The listing builds one solid part. Answer for the finished solid, in the listing's coordinates (mm). A direction names the side the tool comes from. Coordinates: 2 decimals unless noted, no trailing zeros. Write each loop counter-clockwise with the first axis right and the second up, starting at its lowest first coordinate (ties: lowest second). Pieces come first, ordered by that corner, then holes.
from build123d import *

# Parameters (mm, degrees)
SKETCH1_W           = 16
SKETCH1_H           = 37
SKETCH1_W_2         = 13
SKETCH1_H_2         = 34
BOSS_EXTRUDE1_DEPTH = 5
SKETCH2_W           = 16
SKETCH2_H           = 37
BOSS_EXTRUDE2_DEPTH = 1
SKETCH3_W           = 10
SKETCH3_H           = 5
CUT_EXTRUDE1_DEPTH  = 21
SKETCH4_W           = 7
SKETCH4_H           = 2.2
CUT_EXTRUDE2_DEPTH  = 2
SKETCH5_R           = 2.5
CUT_EXTRUDE3_DEPTH  = 2
SKETCH6_W           = 10
SKETCH6_H           = 3
CUT_EXTRUDE4_DEPTH  = 2
CHAMFER1_SIZE       = 1
SKETCH7_W           = 12
SKETCH7_H           = 1
BOSS_EXTRUDE3_DEPTH = 6
SKETCH8_W           = 12
SKETCH8_H           = 1
BOSS_EXTRUDE4_DEPTH = 6
FILLET1_R           = 2
SKETCH9_R           = 1.5
CUT_EXTRUDE5_DEPTH  = 6
SKETCH12_R          = 4
CUT_EXTRUDE6_DEPTH  = 0.8
CHAMFER2_SIZE       = 1.5


with BuildPart() as part:
    # Sketch1 → Boss-Extrude1 (new body)
    with BuildSketch(Plane(origin=(0, 0, 0), x_dir=(1, 0, 0), z_dir=(0, 1, 0))):
        Rectangle(SKETCH1_W, SKETCH1_H)
        Rectangle(SKETCH1_W_2, SKETCH1_H_2, mode=Mode.SUBTRACT)
    extrude(amount=BOSS_EXTRUDE1_DEPTH)

    # Sketch2 → Boss-Extrude2 (add)
    with BuildSketch(Plane.XZ):
        Rectangle(SKETCH2_W, SKETCH2_H)
    extrude(amount=BOSS_EXTRUDE2_DEPTH)

    # Sketch3 → Cut-Extrude1 (cut)
    with BuildSketch(Plane(origin=(8, 0, 0), x_dir=(0, 0, -1), z_dir=(1, 0, 0))):
        with Locations((-11.5, 2.5)):
            Rectangle(SKETCH3_W, SKETCH3_H)
    extrude(amount=-CUT_EXTRUDE1_DEPTH, mode=Mode.SUBTRACT)

    # Sketch4 → Cut-Extrude2 (cut)
    with BuildSketch(Plane.ZY.offset(8)):
        with Locations((-2.4, 3.9)):
            Rectangle(SKETCH4_W, SKETCH4_H)
    extrude(amount=-CUT_EXTRUDE2_DEPTH, mode=Mode.SUBTRACT)

    # Sketch5 → Cut-Extrude3 (cut)
    with BuildSketch(Plane.XY.offset(18.5)):
        with Locations((0, 5.5)):
            Circle(SKETCH5_R)
    extrude(amount=-CUT_EXTRUDE3_DEPTH, mode=Mode.SUBTRACT)

    # Sketch6 → Cut-Extrude4 (cut)
    with BuildSketch(Plane.XY.offset(-17)):
        with Locations((0, 3.5)):
            Rectangle(SKETCH6_W, SKETCH6_H)
    extrude(amount=-CUT_EXTRUDE4_DEPTH, mode=Mode.SUBTRACT)

    # Chamfer1
    chamfer1_edges = [part.edges().sort_by_distance(p)[0] for p in [
        (0, 2, -18.5),
    ]]
    chamfer(chamfer1_edges, length=CHAMFER1_SIZE)

    # Sketch7 → Boss-Extrude3 (add)
    with BuildSketch(Plane(origin=(8, 0, 0), x_dir=(0, 0, -1), z_dir=(1, 0, 0))):
        with Locations((-12.5, -0.5)):
            Rectangle(SKETCH7_W, SKETCH7_H)
    extrude(amount=BOSS_EXTRUDE3_DEPTH)

    # Sketch8 → Boss-Extrude4 (add)
    with BuildSketch(Plane.ZY.offset(8)):
        with Locations((12.5, -0.5)):
            Rectangle(SKETCH8_W, SKETCH8_H)
    extrude(amount=BOSS_EXTRUDE4_DEPTH)

    # Fillet1
    fillet1_edges = [part.edges().sort_by_distance(p)[0] for p in [
        (14, -0.5, 18.5),
        (14, -0.5, 6.5),
        (-14, -0.5, 18.5),
        (-14, -0.5, 6.5),
    ]]
    fillet(fillet1_edges, radius=FILLET1_R)

    # Sketch9 → Cut-Extrude5 (cut)
    with BuildSketch(Plane(origin=(0, 0, 0), x_dir=(1, 0, 0), z_dir=(0, 1, 0))):
        with Locations(Location((-9.25, -11.2, 0), (0, 0, 270))):
            Circle(SKETCH9_R)
        with Locations(Location((9.75, -11.2, 0), (0, 0, 270))):
            Circle(SKETCH9_R)
    extrude(amount=-CUT_EXTRUDE5_DEPTH, mode=Mode.SUBTRACT)

    # Sketch12 → Cut-Extrude6 (cut)
    with BuildSketch(Plane(origin=(0, 0, 17), x_dir=(-1, 0, 0), z_dir=(0, 0, -1))):
        with Locations((0, 5.5)):
            Circle(SKETCH12_R)
    extrude(amount=-CUT_EXTRUDE6_DEPTH, mode=Mode.SUBTRACT)

    # Chamfer2
    chamfer2_edges = [part.edges().sort_by_distance(p)[0] for p in [
        (6.5, 2.5, 6.5),
        (-6.5, 2.5, 6.5),
    ]]
    chamfer(chamfer2_edges, length=CHAMFER2_SIZE - 0.0001)  # a hair under: the kernel refuses the full size


solid = part.part
1. Flat-ended cylindrical pins translate along their axes: P1, Ø8.5, axis at x = 0, z = -3.5, coming from the +Y side; P2, Ø1.8, axis at y = 1.5, z = -7.5, coming from the +X side; P3, Ø1.1, axis at x = -10.5, y = -0.5, coming from the -Z side. Find the tip coordinate at first contact, or state that the pin passes through.
Results found:
P1: stops at y = 0
P2: stops at x = 8
P3: stops at z = 6.5
2. Find the intervals of material crossed by L1, parallel to X at y = -0.25, z = 11.2; L2, parallel to X at y = 0.25, z = -2.5; L3, parallel to Z at x = 1, y = 0.25, in increasing order.
Results found:
L1: x = -14 to -10.75, -7.75 to 8.25, 11.25 to 14
L2: x = -8 to -6.5, 6.5 to 8
L3: z = -18.5 to -17, 17 to 18.5
3. A tool of negligible diameter and unlimited length cuts with its end or side. For faces 4 (the flat face through (-7, 2.8, -2)), 5 (the flat face through (-8, 3, 17)), 6 (the flat face through (0, 1, -17)), 7 (the flat face through (7, 2, 16.5)), from which of +Z, -Z, +X, -X, +Y, -Y can it reach the whole face along a straight path? Write none if from no direction.
Results found:
face 4: -X, +Y
face 5: +Z, -Z, -X, +Y
face 6: +Y
face 7: +X, -X, +Y
4. Section D-D on y = 3.5 is taken. State how many separate pieces and enclosed holes the cut face has, then the cut area to 3 significant figures.
Results found:
separate pieces: 5
enclosed holes: 0
area: 84.6 mm2
5. Section A-A on z = 11.2 is taken. Give the vertices of the cut face in (x, y).
Results found:
outline: (-14, -1) - (-10.75, -1) - (-10.75, 0) - (-14, 0) - close; (-7.75, -1) - (8.25, -1) - (8.25, 0) - (-7.75, 0) - close; (11.25, -1) - (14, -1) - (14, 0) - (11.25, 0) - close
6. Section B-B on x = 9.75 is taken. Give the vertices of the cut face in (y, z), then the cut area to 3 significant figures.
Results found:
outline: (-1, 6.5) - (0, 6.5) - (0, 9.7) - (-1, 9.7) - close; (-1, 12.7) - (0, 12.7) - (0, 18.5) - (-1, 18.5) - close
area: 9.00 mm2
7. For a pull along Z with two mould halves and no side action, classify faces 1 (the flat face through (7.3, 2.5, 5.8)), 2 (the cylindrical face through (-13.4, -0.49, 7.07)), 3 (the flat face through (-5, 3, -18)) as pulls with the +Z half, pulls with the -Z half, needs draft (parallel to the pull), parting line crosses it, or undercut.
Results found:
face 1: undercut
face 2: pulls with the -Z half
face 3: needs draft
